```python
from build123d import *

# Parameters (mm, degrees)
TUBE_R          = 14
TUBE_R_2        = 11.2
TUBE_DEPTH      = 12
SKETCH001_W     = 4
SKETCH001_H     = 8.5
CHAMFER_SIZE    = 0.8
SKETCH_R        = 12.145698
SKETCH_R_2      = 9
PAD_DEPTH       = 2
CHAMFER001_SIZE = 0.5


with BuildPart() as part:
    # Tube → Tube (new body)
    with BuildSketch(Plane.XY):
        Circle(TUBE_R)
        Circle(TUBE_R_2, mode=Mode.SUBTRACT)
    extrude(amount=TUBE_DEPTH)

    # Sketch001 → Groove (revolve, cut)
    with BuildSketch(Plane.YZ):
        with Locations((-15, 5.75)):
            Rectangle(SKETCH001_W, SKETCH001_H)
    revolve(axis=Axis((0, 0, 0), (0, 0, 1)), mode=Mode.SUBTRACT)

    # Chamfer
    chamfer_edges = [part.edges().sort_by_distance(p)[0] for p in [
        (-14, 0, 10),
        (-14, 0, 1.5),
    ]]
    chamfer(chamfer_edges, length=CHAMFER_SIZE)

    # Sketch (on Face7 of Chamfer) → Pad (new body)
    with BuildSketch(Plane(origin=(0, 0, 0), x_dir=(1, 0, 0), z_dir=(0, 0, -1))):
        Circle(SKETCH_R)
        Circle(SKETCH_R_2, mode=Mode.SUBTRACT)
    extrude(amount=-PAD_DEPTH)

    # Chamfer001
    chamfer001_edges = [part.edges().sort_by_distance(p)[0] for p in [
        (-11.2, 0, 12),
    ]]
    chamfer(chamfer001_edges, length=CHAMFER001_SIZE)


solid = part.part
```
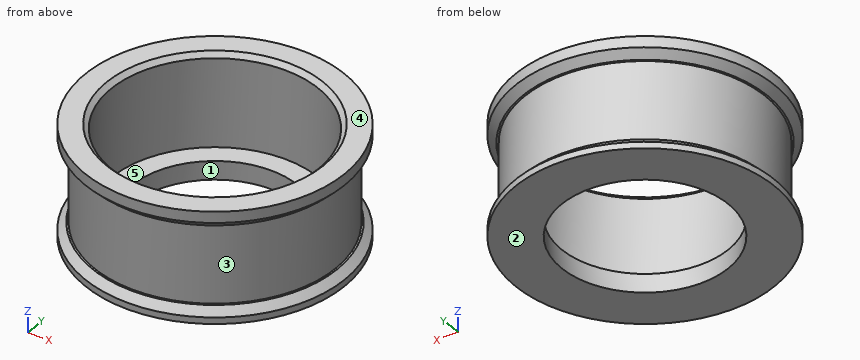
The model under review builds one solid part; all positions refer to its coordinate system, in mm. Face numbers are marked on the shaded views. A direction names the side the tool comes from. Give positions to 0.01 mm unless a question says otherwise; leave off trailing zeros. Write each loop counter-clockwise with the first axis right and the second up, starting at its lowest first coordinate (ties: lowest second). Pieces come first, ordered by that corner, then holes. Notation, with made-up numbers: M 25,64 L 32,64 A14 cw 32,86 Z; hole C -1,49 d3. An arc over 180 degrees is marked long. Write each question's results on one line, items separated by ' | '. Start each with the question number.
1. Mouldability with a two-part tool opening along X and no side actions: class the marked faces 1, 2 and 3 as released by +X, released by -X, zero draft, split by the parting line, or undercut.
2. For the marked faces 4 and 5, list the 3-axis set-ups (+Z, -Z, +X, -X, +Y, -Y) from which the entire face can be reached by the end or side of a thin tool; tool diameter is ignored.
3. Insertion check: pin 1 Ø1 at (x, z) = (4, 4) entering from +Y; pin 2 Ø1.5 at (x, z) = (1, 7) entering from -Y; pin 3 Ø8 at (x, y) = (0.5, -1) entering from +Z; pin 4 Ø6 at (x, z) = (-10.5, 10) entering from +Y. Each pin has a flat end and moves straight along its axis. Give the tip position at first contact, or say it passes through.
4. We need section A-A (x = 0). Write out the cut boundary in (y, z).
5. For probe 1 along X at (y, z) = (0, 8); probe 2 along X at (y, z) = (0, 0.55), list the stretches that pass through material, from the lowest coordinate up. Write a range as [from, to].
6. We need section C-C (z = 2.75). Write out the cut boundary in (x, y), and give its area (3 significant figures).
Results found:
1) face 1: undercut | face 2: zero draft | face 3: split by the parting line
2) face 4: +Z, +X, -X, +Y, -Y | face 5: +Z
3) pin 1: stops at y = 12.52 | pin 2: stops at y = -13 | pin 3: passes through | pin 4: stops at y = 11.75
4) outline: M -14,0 L -9,0 L -9,2 L -11.2,2 L -11.2,11.5 L -11.7,12 L -14,12 L -14,10.8 L -13.2,10 L -13,10 L -13,1.5 L -13.2,1.5 L -14,0.7 Z; M 9,0 L 14,0 L 14,0.7 L 13.2,1.5 L 13,1.5 L 13,10 L 13.2,10 L 14,10.8 L 14,12 L 11.7,12 L 11.2,11.5 L 11.2,2 L 9,2 Z
5) probe 1: x = [-13, -11.2], [11.2, 13] | probe 2: x = [-14, -9], [9, 14]
6) outline: C 0,0 d26; hole C 0,0 d22.4 | area: 137 mm^2
